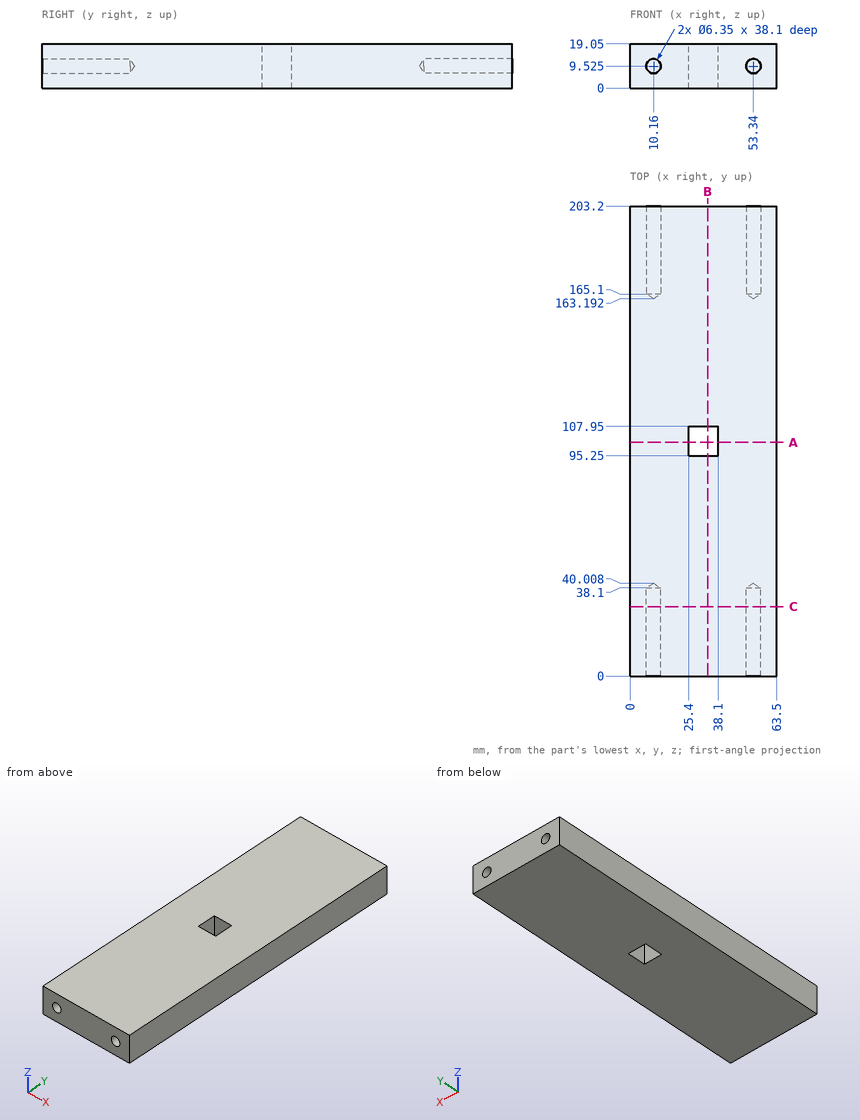
Here's the drawing with two shaded views (mm, measured from the low corner). I have some questions. Coordinates: 2 decimals unless noted, no trailing zeros. Write each loop counter-clockwise with the first axis right and the second up, starting at its lowest first coordinate (ties: lowest second). Pieces come first, ordered by that corner, then holes. Notation, with made-up numbers: M 28.25,-25 L 33.25,-25 A24 cw 33.25,-8 Z; hole C 9.25,-14.75 d4. An arc over 180 degrees is marked long. Answer as CSV lines item,"result". Start each with the question number.
1) For P1, Ø8, axis at x = 8.5, y = 36, coming from the -Z side; P2, Ø5.5, axis at x = 10.16, z = 9.525, coming from the -Y side (1 decimal); P3, Ø4, axis at x = 53.34, z = 9.525, coming from the +Y side, each with a flat end and sliding along its axis, tell me the tip position at first contact or that it passes through.
2) I want a section at B-B, the plane x = 33.5. Please give me the cut outline in (y, z).
3) I want a section at A-A, the plane y = 101. Please give me the cut outline in (x, z).
4) Please list where these lines run through material, in increasing order: line 1 (Z direction, x = 53.34, y = 191.5); line 2 (Y direction, x = 31, z = 3.75); line 3 (X direction, y = 15.5, z = 8.5) (1 decimal). Write a range as from..to.
5) I want a section at C-C, the plane y = 30. Give the number of separate pieces and of enclosed holes in the cut face, and give its area (3 significant figures).
Data:
1,P1,"stops at z = 0"
1,P2,"stops at y = 38.4"
1,P3,"stops at y = 164.39"
2,outline,"M 0,0 L 95.25,0 L 95.25,19.05 L 0,19.05 Z; M 107.95,0 L 203.2,0 L 203.2,19.05 L 107.95,19.05 Z"
3,outline,"M 0,0 L 25.4,0 L 25.4,19.05 L 0,19.05 Z; M 38.1,0 L 63.5,0 L 63.5,19.05 L 38.1,19.05 Z"
4,line 1,"z = 0..6.35, 12.7..19.05"
4,line 2,"y = 0..95.25, 107.95..203.2"
4,line 3,"x = 0..7.2, 13.2..50.3, 56.3..63.5"
5,separate pieces,"1"
5,enclosed holes,"2"
5,area,"1,150 mm^2"
